Answer from the drawing. Dimensions are ordinates in mm from the lowest x, y and z of the part. A direction names the side the tool comes from. Round coordinates to 2 decimals unless told otherwise and drop trailing zeros. Write each loop counter-clockwise with the first axis right and the second up, starting at its lowest first coordinate (ties: lowest second). Pieces come first, ordered by that corner, then holes. Notation, with made-up numbers: (67, -19) - (102, -19) arc R21 cw to (102, 17) - close; hole circle Ø9 at (50.25, -7). An arc over 180 degrees is marked (long way). Use a Markdown table: item, result. Add a question column.
1) Each of these flat-tipped pins is pushed along its axis until it touches: P1, Ø2, axis at y = 67.5, z = 9, coming from the -X side; P2, Ø1, axis at x = 29.5, z = 3.5, coming from the +Y side; P3, Ø1, axis at x = 14, z = 1, coming from the -Y side; P4, Ø24, axis at x = 43, y = 43, coming from the -Z side. Where does it stop, or does it pass through?
2) A tool of negligible diameter and unlimited length cuts with its end or side. For the marked faces 3 and 4, from which of +Z, -Z, +X, -X, +Y, -Y can it reach the whole face along a straight path? Write none if from no direction.
3) Find the intervals of material crossed by probe 1 along Y at (x, z) = (43, 6.15); probe 2 along Z at (x, y) = (61.5, 60); probe 3 along X at (y, z) = (40, 1), in increasing order. Write a range as from..to.
4) A cutting plane is placed at C-C (z = 1.75). Give the vertices of the cut face in (x, y), then the cut area to 3 significant figures.
5) Determine the mould class of the marked faces 1 and 2 for opening direction X: +X half, -X half, draft (parallel to the pull), parting line (faces both ways), or undercut.
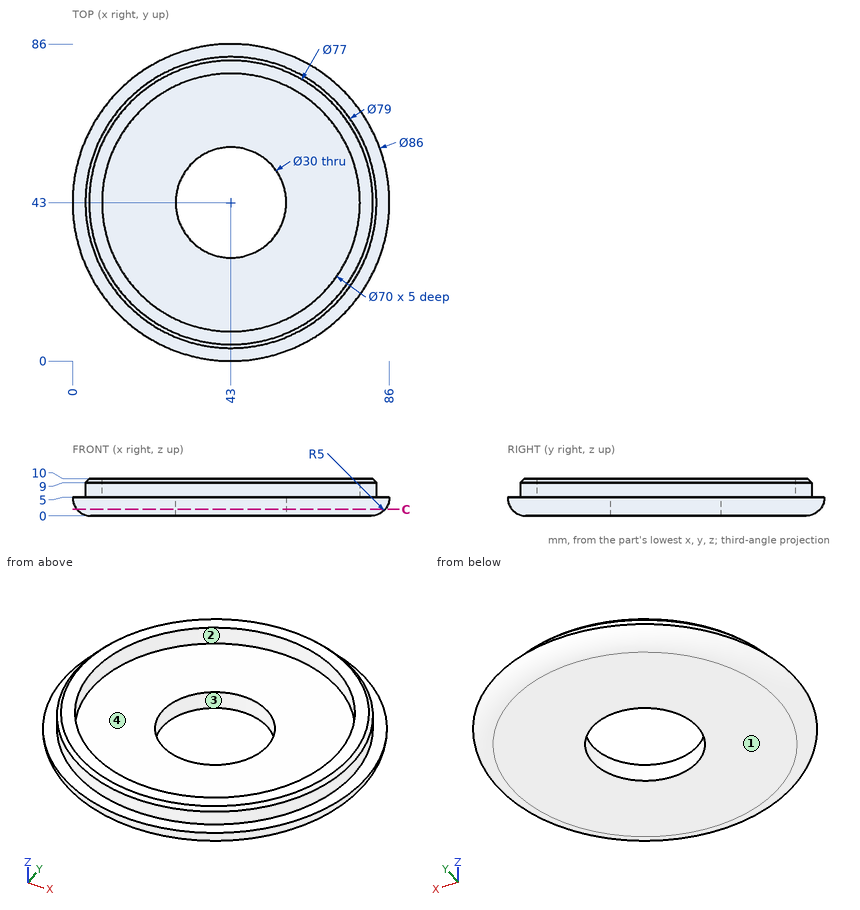
Entries:
| question | item | result |
|---|---|---|
| 1 | P1 | stops at x = 11.25 |
| 1 | P2 | stops at y = 83.8 |
| 1 | P3 | stops at y = 13.06 |
| 1 | P4 | passes through |
| 2 | face 3 | +Z, -Z |
| 2 | face 4 | +Z |
| 3 | probe 1 | y = 3.5..8, 78..82.5 |
| 3 | probe 2 | z = 0..5 |
| 3 | probe 3 | x = 2.11..28.3, 57.7..83.89 |
| 4 | outline | circle Ø83.6 at (43, 43); hole circle Ø30 at (43, 43) |
| 4 | area | 4,780 mm² |
| 5 | face 1 | draft |
| 5 | face 2 | undercut |
